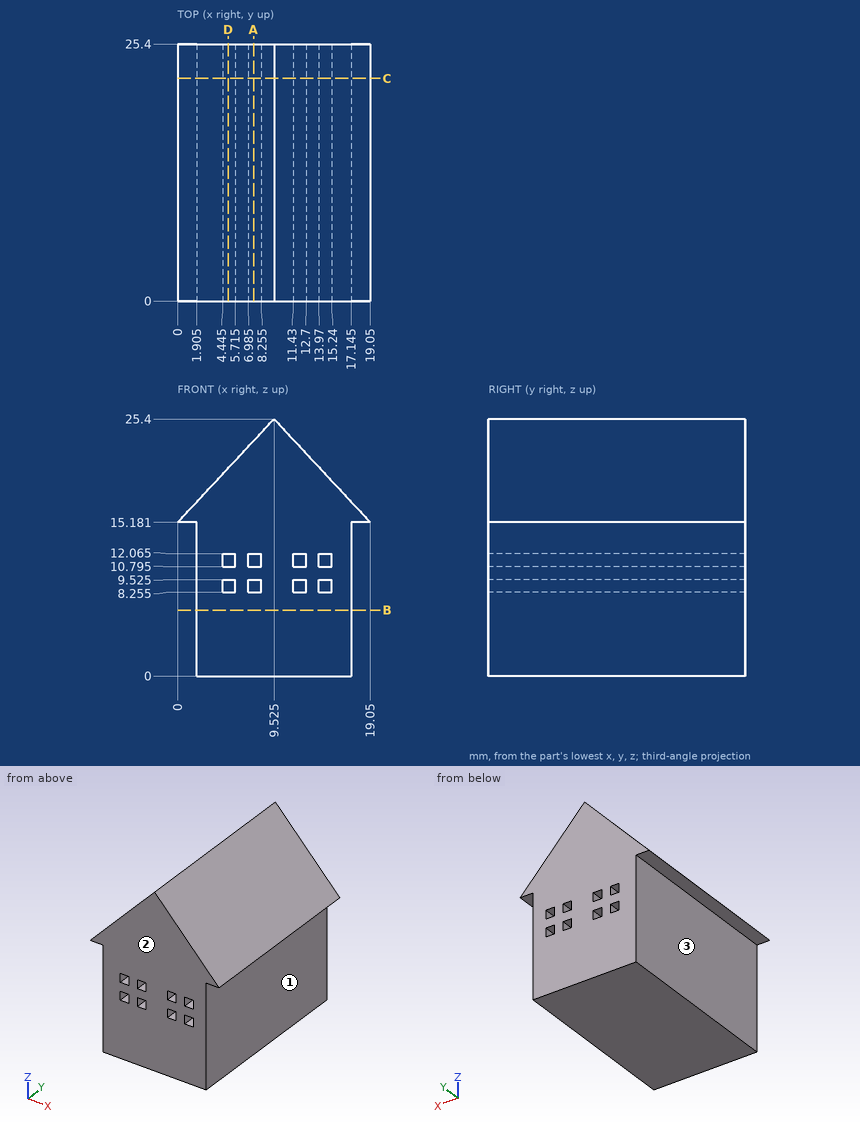
Job drawing, mm, ordinate dimensions from the low corner. One solid piece. A direction names the side the tool comes from. Round coordinates to 2 decimals unless told otherwise and drop trailing zeros. Loops run counter-clockwise (first coordinate to the right, second up) from the corner with the lowest first, then second, coordinate; pieces in that order, holes last. Notation, with made-up numbers: (-33.75, -5) -> (-25.75, -5) arc R4 ccw to (-25.75, -1) -> close; hole circle Ø3 at (39, -38). An arc over 180 degrees is marked (long way). Use CSV: the item, a comma, the result in double quotes. Start each with the question number.
Q1. Flat gauge pins, fed straight in: pin 1 Ø2 at (x, y) = (3.5, 15) entering from +Z; pin 2 Ø0.6 at (y, z) = (13, 11.5) entering from -X (3 decimals); pin 3 Ø1 at (y, z) = (16.5, 8.5) entering from +X (3 decimals). Where does each tip first touch, or does it go through?
Q2. Drill centre lines: L1, parallel to X at y = 18, z = 11.5 (1 decimal); L2, parallel to X at y = 9.5, z = 3 (1 decimal); L3, parallel to Z at x = 8, y = 8.75 (1 decimal). Where is each one in solid material? Low to high.
Q3. Which spindle directions (+Z, -Z, +X, -X, +Y, -Y) get a long thin tool onto all of the face, cutting with end or side? Do the marked faces 1, 2 and 3. Say none if no direction does.
Q4. Saw through at A-A on x = 7.5. Give the cut face in (y, z) (1 decimal).
Q5. Saw through at D-D on x = 5. Give the cut face in (y, z) (1 decimal).
Q6. Saw through at B-B on z = 6.5. Give the cut face in (x, y) (1 decimal).
Q7. Saw through at C-C on y = 22. Count the separate pieces of the cut face and the enclosed holes in it, and give its area (3 significant figures).
Solutions:
1,pin 1,"stops at z = 20.01"
1,pin 2,"stops at x = 1.905"
1,pin 3,"stops at x = 17.145"
2,L1,"x = 1.9 to 4.4, 5.7 to 7, 8.3 to 11.4, 12.7 to 14, 15.2 to 17.1"
2,L2,"x = 1.9 to 17.1"
2,L3,"z = 0 to 8.3, 9.5 to 10.8, 12.1 to 23.8"
3,face 1,"-Z, +X, +Y, -Y"
3,face 2,"+Z, -Z, +X, -X, -Y"
3,face 3,"-Z, -X, +Y, -Y"
4,outline,"(0, 0) -> (25.4, 0) -> (25.4, 8.3) -> (0, 8.3) -> close; (0, 9.5) -> (25.4, 9.5) -> (25.4, 10.8) -> (0, 10.8) -> close; (0, 12.1) -> (25.4, 12.1) -> (25.4, 23.2) -> (0, 23.2) -> close"
5,outline,"(0, 0) -> (25.4, 0) -> (25.4, 8.3) -> (0, 8.3) -> close; (0, 9.5) -> (25.4, 9.5) -> (25.4, 10.8) -> (0, 10.8) -> close; (0, 12.1) -> (25.4, 12.1) -> (25.4, 20.5) -> (0, 20.5) -> close"
6,outline,"(1.9, 0) -> (17.1, 0) -> (17.1, 25.4) -> (1.9, 25.4) -> close"
7,separate pieces,"1"
7,enclosed holes,"8"
7,area,"316 mm^2"
